Geometry check sheet. Reference: the model listing, model coordinates, mm. Face numbers are marked on the shaded views. Coordinates: 2 decimals unless noted, no trailing zeros. Write each loop counter-clockwise with the first axis right and the second up, starting at its lowest first coordinate (ties: lowest second). Pieces come first, ordered by that corner, then holes. Notation, with made-up numbers: (77, -37) -> (96, -37) arc R14 ccw to (96, -29) -> close; hole circle Ø3 at (5.5, -37.75). An arc over 180 degrees is marked (long way). One line per question, with ' | ' between items.
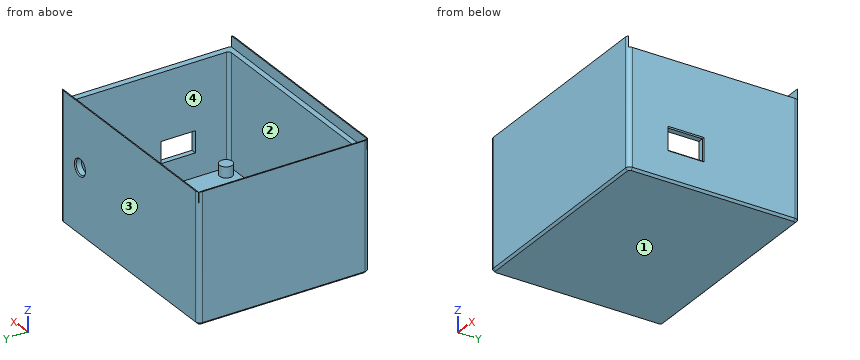
Autodesk Fusion 360 part; units mm, degrees
sketch "Sketch1" plane through (0, 0, 0) normal (0, 0, 1) x (1, 0, 0)
  line L0 (48, 40) -> (-48, 40)
  line L1 (-50, 38) -> (-50, -38)
  line L2 (-48, -40) -> (48, -40)
  line L3 (50, -38) -> (50, 38)
  line L4 (50, 40) -> (-50, -40) construction
  line L5 (-50, 40) -> (50, -40) construction
  line L6 (45.5, 37) -> (-45.5, 37)
  line L7 (-47, 35.5) -> (-47, -35.5)
  line L8 (-45.5, -37) -> (45.5, -37)
  line L9 (47, -35.5) -> (47, 35.5)
  line L10 (47, 37) -> (-47, -37) construction
  line L11 (-47, 37) -> (47, -37) construction
  arc A0 (-48, 40) -> (-50, 38) centre (-48, 38) ccw
  arc A1 (50, 38) -> (48, 40) centre (48, 38) ccw
  arc A2 (48, -40) -> (50, -38) centre (48, -38) ccw
  arc A3 (-50, -38) -> (-48, -40) centre (-48, -38) ccw
  arc A4 (-45.5, 37) -> (-47, 35.5) centre (-45.5, 35.5) ccw
  arc A5 (47, 35.5) -> (45.5, 37) centre (45.5, 35.5) ccw
  arc A6 (45.5, -37) -> (47, -35.5) centre (45.5, -35.5) ccw
  arc A7 (-47, -35.5) -> (-45.5, -37) centre (-45.5, -35.5) ccw
  dimension "d1" = 100
  dimension "d2" = 80
  dimension "d3" = 94
  dimension "d4" = 74
  dimension "d5" = 2
  dimension "d6" = 1.5
extrude "Extrude1" add sketch "Sketch1" along normal blind 55
extrude "Extrude2" add sketch "Sketch1" along normal blind 3 contours L6 L7 L8 L9 A4 A5 A6 A7
chamfer "Chamfer1" distance 1 angle 45 8 edges at (50, 0, 0) (49.4142, 39.4142, 0) (0, 40, 0) (-49.4142, 39.4142, 0) (-50, 0, 0) (-49.4142, -39.4142, 0) (0, -40, 0) (49.4142, -39.4142, 0)
sketch "Sketch2" plane through (0, 0, 3) normal (0, 0, 1) x (-1, 0, 0)
  arc A0 (47, 35.5) -> (45.5, 37) centre (45.5, 35.5) ccw
  line L0 (45.5, 37) -> (-45.5, 37)
  arc A1 (-45.5, 37) -> (-47, 35.5) centre (-45.5, 35.5) ccw
  line L1 (-47, 35.5) -> (-47, -35.5)
  arc A2 (-47, -35.5) -> (-45.5, -37) centre (-45.5, -35.5) ccw
  line L2 (-45.5, -37) -> (45.5, -37)
  arc A3 (45.5, -37) -> (47, -35.5) centre (45.5, -35.5) ccw
  line L3 (47, -35.5) -> (47, 35.5)
  circle A4 centre (42.5, -32.5) radius 3
  line L4 (50, 0) -> (-50, 0) construction
  line L5 (0, -40) -> (0, 40) construction
  circle A5 centre (42.5, 32.5) radius 3
  circle A6 centre (-42.5, -32.5) radius 3
  circle A7 centre (-42.5, 32.5) radius 3
  dimension "d12" = 6
  dimension "d13" = 4.5
  dimension "d14" = 4.5
extrude "Extrude3" add sketch "Sketch2" along normal blind 5 contours A4 | A5 | A6 | A7
sketch "Sketch3" plane through (50, 0, 0) normal (1, 0, 0) x (0, 1, 0)
  line L0 (-38, 1) -> (38, 1)
  line L1 (38, 1) -> (38, 55)
  line L2 (38, 55) -> (-38, 55)
  line L3 (-38, 55) -> (-38, 1)
  line L4 (-5, 24) -> (-21, 24)
  line L5 (-21, 24) -> (-21, 14)
  line L6 (-21, 14) -> (-5, 14)
  line L7 (-5, 14) -> (-5, 24)
  line L8 (-5, 24) -> (-21, 14) construction
  line L9 (-21, 24) -> (-5, 14) construction
  point P0 (-13, 19)
  dimension "d17" = 16
  dimension "d18" = 10
  dimension "d19" = 25
  dimension "d20" = 18
extrude "Extrude4" cut sketch "Sketch3" against normal blind 3 contours L4 L5 L6 L7
sketch "Sketch4" plane through (0, 40, 0) normal (0, 1, 0) x (-1, 0, 0)
  line L0 (-48, 1) -> (48, 1)
  line L1 (48, 1) -> (48, 55)
  line L2 (48, 55) -> (-48, 55)
  line L3 (-48, 55) -> (-48, 1)
  circle A0 centre (-36, 31) radius 3.5
  dimension "d23" = 7
  dimension "d24" = 12
  dimension "d25" = 30
extrude "Extrude5" cut sketch "Sketch4" against normal blind 3 contours A0
extrude "Extrude6" add 1 faces at (-15.1667, 39, 55) along direction (0, 0, 1) blind 5
sketch "Sketch5" plane through (0, 0, 60) normal (0, 0, 1) x (-1, 0, 0)
  arc A0 (47, 35.5) -> (45.5, 37) centre (45.5, 35.5) ccw
  line L0 (47, 35.5) -> (47, -35.5)
  arc A1 (45.5, -37) -> (47, -35.5) centre (45.5, -35.5) ccw
  line L1 (45.5, -37) -> (-45.5, -37)
  arc A2 (-47, -35.5) -> (-45.5, -37) centre (-45.5, -35.5) ccw
  line L2 (-47, -35.5) -> (-47, 35.5)
  arc A3 (-45.5, 37) -> (-47, 35.5) centre (-45.5, 35.5) ccw
  line L3 (-45.5, 37) -> (45.5, 37)
  arc A4 (50, 38) -> (48, 40) centre (48, 38) ccw
  line L4 (48, 40) -> (-48, 40)
  arc A5 (-48, 40) -> (-50, 38) centre (-48, 38) ccw
  line L5 (-50, 38) -> (-50, -38)
  arc A6 (-50, -38) -> (-48, -40) centre (-48, -38) ccw
  line L6 (-48, -40) -> (48, -40)
  arc A7 (48, -40) -> (50, -38) centre (48, -38) ccw
  line L7 (50, -38) -> (50, 38)
  line L8 (49.5, 39.5) -> (-49.5, 39.5)
  line L9 (-49.5, 39.5) -> (-49.5, -39.5)
  line L10 (-49.5, -39.5) -> (49.5, -39.5)
  line L11 (49.5, -39.5) -> (49.5, 39.5)
  line L12 (46.3, 36.3) -> (-46.3, 36.3)
  line L13 (-46.3, 36.3) -> (-46.3, -36.3)
  line L14 (-46.3, -36.3) -> (46.3, -36.3)
  line L15 (46.3, -36.3) -> (46.3, 36.3)
  dimension "d30" = 0.5
  dimension "d31" = 0.5
  dimension "d32" = 0.5
  dimension "d33" = 0.5
  dimension "d34" = 3.2
  dimension "d35" = 3.2
  dimension "d36" = 3.2
  dimension "d37" = 3.2
extrude "Extrude7" cut sketch "Sketch5" against normal blind 5 contours A0 L0 A1 L1 A2 L2 A3 L3 | A4 A5 A6 A7 L8 L9 L10 L11
extrude "Extrude8" cut 1 faces at (49.6667, 12.6667, 60) along direction (0, 0, -1) blind 5
chamfer "Chamfer2" distance 0.5 angle 45 4 edges at (50, -5, 19) (50, -13, 24) (50, -21, 19) (50, -13, 14)
chamfer "Chamfer3" distance 0.5 angle 45 1 edges at (39.2631, 40, 32.2657)
1. Material ranges on line 1 (Z direction, x = 36, y = 37.75); line 2 (X direction, y = -18.5, z = 13); line 3 (Y direction, x = 4.5, z = 23), recorded low to high. Write a range as from..to.
Worked answers:
line 1: 0..27.5, 34.5..55 | line 2: -50..-47, 47..50 | line 3: -40..-37, 37..40
2. Mould release check, pull along Y, two halves, no side actions. Record for the marked faces 1, 2, 3 and 4: released by +Y, released by -Y, zero draft, split by the parting line, or undercut.
Worked answers:
face 1: zero draft | face 2: undercut | face 3: released by +Y | face 4: undercut
3. Cross-section at C-C on x = -42.5. Record the boundary of the cut face in (y, z).
Worked answers:
outline: (-40, 1) -> (-39, 0) -> (39, 0) -> (40, 1) -> (40, 60) -> (39.5, 60) -> (39.5, 55) -> (37, 55) -> (37, 3) -> (35.5, 3) -> (35.5, 8) -> (29.5, 8) -> (29.5, 3) -> (-29.5, 3) -> (-29.5, 8) -> (-35.5, 8) -> (-35.5, 3) -> (-37, 3) -> (-37, 55) -> (-39.5, 55) -> (-39.5, 60) -> (-40, 60) -> close
4. Cross-section at B-B on z = 52.5. Record the boundary of the cut face in (x, y), and give its area (3 significant figures).
Worked answers:
outline: (-50, -38) arc R2 ccw to (-48, -40) -> (48, -40) arc R2 ccw to (50, -38) -> (50, 38) arc R2 ccw to (48, 40) -> (-48, 40) arc R2 ccw to (-50, 38) -> close; hole (-47, -35.5) arc R1.5 ccw to (-45.5, -37) -> (45.5, -37) arc R1.5 ccw to (47, -35.5) -> (47, 35.5) arc R1.5 ccw to (45.5, 37) -> (-45.5, 37) arc R1.5 ccw to (-47, 35.5) -> close | area: 1,040 mm²
5. Go/stop test with flat-tipped pins: P1, Ø4, axis at x = -19.5, y = 18.5, coming from the -Z side; P2, Ø3, axis at x = -43.5, y = -32.5, coming from the +Z side; P3, Ø1, axis at x = -1, y = -28.5, coming from the +Z side; P4, Ø1.5, axis at y = 2, z = 57.5, coming from the +X side. Record where each tip stops, or that it passes through.
Worked answers:
P1: z = 0 | P2: z = 8 | P3: z = 3 | P4: x = -49.5
6. Cross-section at A-A on y = -9.5. Record the boundary of the cut face in (x, z).
Worked answers:
outline: (-50, 1) -> (-49, 0) -> (49, 0) -> (50, 1) -> (50, 13.5) -> (49.5, 14) -> (47, 14) -> (47, 3) -> (-47, 3) -> (-47, 55) -> (-49.5, 55) -> (-49.5, 60) -> (-50, 60) -> close; (47, 24) -> (49.5, 24) -> (50, 24.5) -> (50, 55) -> (47, 55) -> close
7. Cross-section at D-D on y = 32.5. Record the boundary of the cut face in (x, z), and give its area (4 significant figures).
Worked answers:
outline: (-50, 1) -> (-49, 0) -> (49, 0) -> (50, 1) -> (50, 55) -> (47, 55) -> (47, 3) -> (45.5, 3) -> (45.5, 8) -> (39.5, 8) -> (39.5, 3) -> (-39.5, 3) -> (-39.5, 8) -> (-45.5, 8) -> (-45.5, 3) -> (-47, 3) -> (-47, 55) -> (-49.5, 55) -> (-49.5, 60) -> (-50, 60) -> close | area: 673.5 mm²
